Here's the drawing with two shaded views (mm, measured from the low corner). I have some questions. A direction names the side the tool comes from. Round coordinates to 2 decimals unless told otherwise and drop trailing zeros. Write each loop counter-clockwise with the first axis right and the second up, starting at its lowest first coordinate (ties: lowest second). Pieces come first, ordered by that corner, then holes.
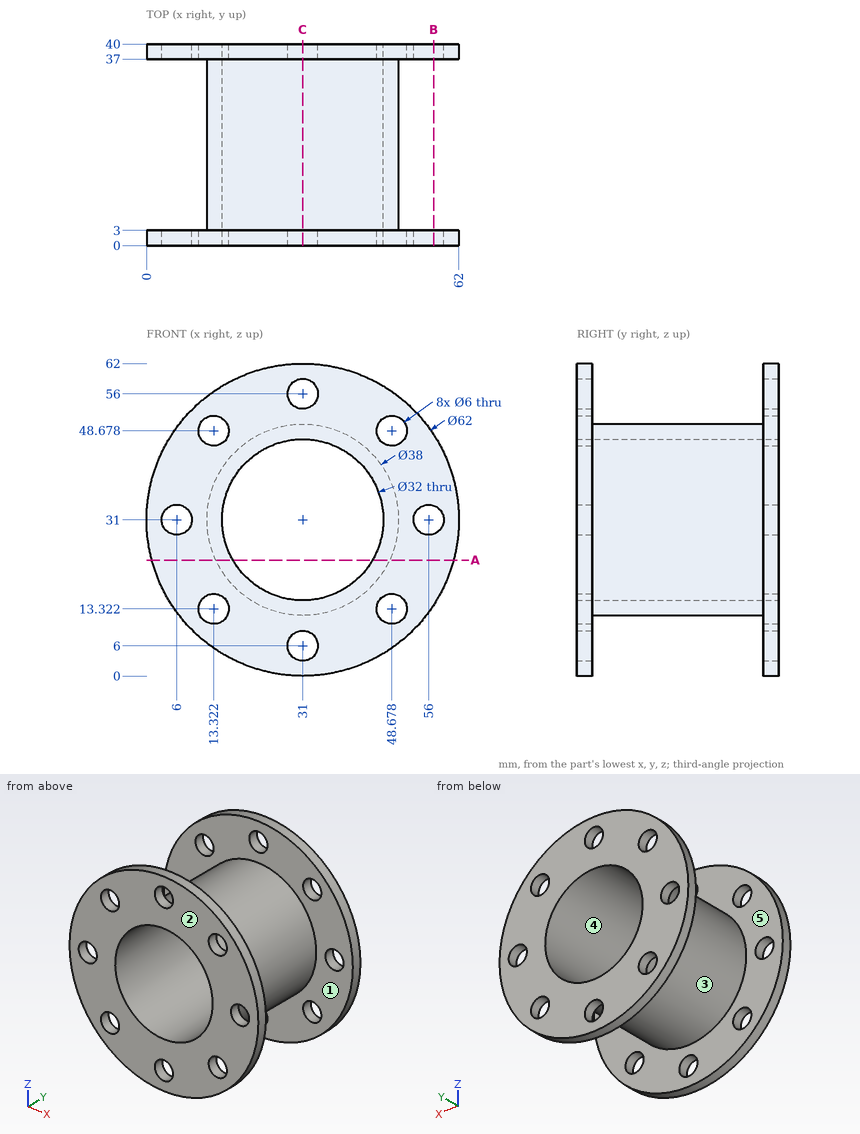
Q1. If I drill on L1, parallel to Y at x = 22.5, z = 10.5; L2, parallel to X at y = 1, z = 31; L3, parallel to X at y = 31, z = 17 (1 decimal), over which ranges is the centre line in solid material (lowest first)?
Q2. Imagine slicing it at B-B, the plane x = 57. Write out the boundary of the cut face in (y, z), then the cut area to 3 significant figures.
Q3. On a 3-axis mill with a long thin cutter (end or side, diameter ignored), from which of +Z, -Z, +X, -X, +Y, -Y can I reach the whole of each face in a straight line? I mean the marked faces 1 and 2. Say none if no direction works.
Q4. Imagine slicing it at A-A, the plane z = 23. Write out the boundary of the cut face in (x, y).
Q5. I'm going to push flat-ended pins straight in: pin 1 Ø10 at (y, z) = (5, 29) entering from -X; pin 2 Ø9.5 at (x, z) = (31, 56) entering from +Y; pin 3 Ø1.5 at (x, y) = (30, 9.5) entering from +Z; pin 4 Ø3 at (y, z) = (34, 46.5) entering from -X (1 decimal). Where does each tip first touch, or does it pass through?
Q6. Imagine slicing it at C-C, the plane x = 31. Count the separate pieces of the cut face and the enclosed holes in it, then the cut area to 3 significant figures.
Q7. We'd pull the mould along X, two halves only. Please class the marked faces 3, 4 and 5: pulls with the +X half, pulls with the -X half, needs draft (parallel to the pull), parting line crosses it, or undercut.
Results found:
1. L1: y = 0 to 3, 37 to 40
1. L2: x = 0 to 3, 9 to 15, 47 to 53, 59 to 62
1. L3: x = 18.2 to 23.3, 38.7 to 43.8
2. outline: (0, 14.12) - (3, 14.12) - (3, 28.17) - (0, 28.17) - close; (0, 33.83) - (3, 33.83) - (3, 47.88) - (0, 47.88) - close; (37, 14.12) - (40, 14.12) - (40, 28.17) - (37, 28.17) - close; (37, 33.83) - (40, 33.83) - (40, 47.88) - (37, 47.88) - close
2. area: 169 mm2
3. face 1: none
3. face 2: +Z, -Z, +X, -X, -Y
4. outline: (1.05, 0) - (17.14, 0) - (17.14, 40) - (1.05, 40) - (1.05, 37) - (13.77, 37) - (13.77, 3) - (1.05, 3) - close; (44.86, 0) - (60.95, 0) - (60.95, 3) - (48.23, 3) - (48.23, 37) - (60.95, 37) - (60.95, 40) - (44.86, 40) - close
5. pin 1: stops at x = 0
5. pin 2: stops at y = 40
5. pin 3: stops at z = 50
5. pin 4: stops at x = 18.2
6. separate pieces: 6
6. enclosed holes: 0
6. area: 312 mm2
7. face 3: parting line crosses it
7. face 4: undercut
7. face 5: needs draft
